```python
from build123d import *

# Parameters (mm, degrees)
F1_DEPTH  = 3.175
F2_W      = 17.018
F2_H      = 8.128
F3_DEPTH  = 1.5875
F5_DEPTH  = 1.5875
F6_W      = 10.05
F6_H      = 8.76
F7_DEPTH  = 3
F8_R      = 3.5
F9_DEPTH  = 3.5
F11_DEPTH = 1.5875


with BuildPart() as f1:
    # F0 (on Top) → F1 (new body)
    with BuildSketch(Plane.XY):
        with BuildLine():
            Line((-12.0608898944, 10.16), (-19.05, 10.16))
            Line((-19.05, 10.16), (-19.05, 0))
            Line((-19.05, 0), (0, 0))
            Line((0, 0), (0, 10.16))
            Line((0, 10.16), (-6.9891101056, 10.16))
            ThreePointArc((-6.9891101056, 10.16), (-7.425, 10.06), (-7.8608898944, 10.16))
            Line((-7.8608898944, 10.16), (-9.0891101056, 10.16))
            ThreePointArc((-9.0891101056, 10.16), (-9.525, 10.06), (-9.9608898944, 10.16))
            Line((-9.9608898944, 10.16), (-11.1891101056, 10.16))
            ThreePointArc((-11.1891101056, 10.16), (-11.625, 10.06), (-12.0608898944, 10.16))
        make_face()
        with BuildLine():
            ThreePointArc((-10.625, 11.06), (-12.1560885546, 11.9073163206), (-12.0608898944, 10.16))
            Line((-12.0608898944, 10.16), (-11.1891101056, 10.16))
            ThreePointArc((-11.1891101056, 10.16), (-10.7776836794, 10.5289114454), (-10.625, 11.06))
        make_face()
        with BuildLine():
            Line((-11.1891101056, 10.16), (-12.0608898944, 10.16))
            ThreePointArc((-12.0608898944, 10.16), (-11.625, 10.06), (-11.1891101056, 10.16))
        make_face()
        with BuildLine():
            ThreePointArc((-8.525, 11.06), (-10.0560885546, 11.9073163206), (-9.9608898944, 10.16))
            Line((-9.9608898944, 10.16), (-9.0891101056, 10.16))
            ThreePointArc((-9.0891101056, 10.16), (-8.6776836794, 10.5289114454), (-8.525, 11.06))
        make_face()
        with BuildLine():
            Line((-9.0891101056, 10.16), (-9.9608898944, 10.16))
            ThreePointArc((-9.9608898944, 10.16), (-9.525, 10.06), (-9.0891101056, 10.16))
        make_face()
        with BuildLine():
            ThreePointArc((-7.8608898944, 10.16), (-7.425, 10.06), (-6.9891101056, 10.16))
            Line((-6.9891101056, 10.16), (-7.8608898944, 10.16))
        make_face()
        with BuildLine():
            Line((-7.8608898944, 10.16), (-6.9891101056, 10.16))
            ThreePointArc((-6.9891101056, 10.16), (-6.5776836794, 10.5289114454), (-6.425, 11.06))
            ThreePointArc((-6.425, 11.06), (-7.9560885546, 11.9073163206), (-7.8608898944, 10.16))
        make_face()
    extrude(amount=F1_DEPTH)

    # F2 (on face) → F3 (cut)
    with BuildSketch(Plane.XY.offset(3.175)):
        with Locations((-9.525, 5.08)):
            Rectangle(F2_W, F2_H)
    extrude(amount=-F3_DEPTH, mode=Mode.SUBTRACT)

    # F4 (on face) → F5 (join, through all)
    with BuildSketch(Plane.XY.offset(1.5875)):
        Polygon((-9.525, 8.5074082457), (-9.525, 9.144), (-10.1615917543, 9.144), (-18.034, 1.6525917543), (-18.034, 1.016), (-17.3974082457, 1.016), (-9.825, 8.2219273099), align=None)
        Polygon((-8.8884082457, 9.144), (-9.525, 9.144), (-9.525, 8.5074082457), (-9.225, 8.2219273099), (-1.6525917543, 1.016), (-1.016, 1.016), (-1.016, 1.6525917543), align=None)
    extrude(amount=F5_DEPTH)

    # F6 (on face) → F7 (join)
    with BuildSketch(Plane(origin=(0, 0, 0), x_dir=(1, 0, 0), z_dir=(0, 0, -1))):
        with Locations((-9.525, -5.08)):
            Rectangle(F6_W, F6_H)
    extrude(amount=F7_DEPTH)

    # F8 (on face) → F9 (cut)
    with BuildSketch(Plane(origin=(0, 0, -3), x_dir=(1, 0, 0), z_dir=(0, 0, -1))):
        with Locations((-9.525, -5.08)):
            Circle(F8_R)
    extrude(amount=-F9_DEPTH, mode=Mode.SUBTRACT)

    # F10 (on face) → F11 (join, through all)
    with BuildSketch(Plane.XY.offset(1.5875)):
        Polygon((-9.525, 8.5074082457), (-9.975, 8.0791868419), (-9.975, 1.016), (-9.525, 1.016), (-9.075, 1.016), (-9.075, 8.0791868419), align=None)
    extrude(amount=F11_DEPTH)


solid = f1.part
```
Here's how the part is built. I have some questions about the finished solid (model axes, mm). A direction names the side the tool comes from. Give positions to 0.01 mm unless a question says otherwise; leave off trailing zeros. Write each loop counter-clockwise with the first axis right and the second up, starting at its lowest first coordinate (ties: lowest second). Pieces come first, ordered by that corner, then holes. Notation, with made-up numbers: (13.5, 3) -> (48.5, 3) arc R15 cw to (48.5, 29) -> close; hole circle Ø6 at (9, 12.25). An arc over 180 degrees is marked (long way). Use one line per item in the form item = value.
1) On a 3-axis mill with a long thin cutter (end or side, diameter ignored), from which of +Z, -Z, +X, -X, +Y, -Y can I reach the whole of each face in a straight line? I mean faces 4 (the face through (-14.55, 5, -1)), 5 (the face through (-12, 8, -3)), 6 (the face through (-5.42, 4.6, 2.37)), 7 (the face through (-4.5, 5, -1)), 8 (the face through (-10, 0.7, -1)). Say none if no direction works.
Verdict:
face_4 = -Z, -X, +Y, -Y
face_5 = -Z, +X, -X, +Y, -Y
face_6 = +Z
face_7 = -Z, +X, +Y, -Y
face_8 = -Z, +X, -X, -Y
2) Suppose I cut it at B-B (x = -3). Please give me the cut outline in (y, z) (1 decimal).
Verdict:
outline = (0, 0) -> (10.2, 0) -> (10.2, 3.2) -> (9.1, 3.2) -> (9.1, 1.6) -> (3.5, 1.6) -> (3.5, 3.2) -> (2.3, 3.2) -> (2.3, 1.6) -> (1, 1.6) -> (1, 3.2) -> (0, 3.2) -> close
3) If I drill on L1, parallel to X at y = 5.08, z = -1.7 (3 decimals); L2, parallel to Z at x = -13.5, y = 2.5; L3, parallel to Y at x = -13.25, z = -2, over which ranges is the centre line in solid material (lowest first)? Write a range as [from, to].
Verdict:
L1 = [-14.55, -13.025], [-6.025, -4.5]
L2 = [-3, 1.59]
L3 = [0.7, 9.46]
4) I'm going to push flat-ended pins straight in: pin 1 (1.6 mm diameter, centred on x = -16.5, z = 2, fed in from +Y); pin 2 (0.6 mm diameter, centred on x = -10.5, z = 2, fed in from +Y); pin 3 (2 mm diameter, centred on x = -5.5, y = 3, fed in from +Z). Where does each tip first touch, or does it pass through?
Verdict:
pin_1 = 10.16
pin_2 = 11.8
pin_3 = 1.59
5) We'd pull the mould along X, two halves only. Please class faces 1 (the face through (-10, 0, 2)), 2 (the face through (0, 5, 2)), 3 (the face through (-3, 7, 1.588)): +X half, -X half, draft (parallel to the pull), parting line (faces both ways), or undercut.
Verdict:
face_1 = draft
face_2 = +X half
face_3 = undercut
6) Suppose I cut it at A-A (z = -2.5). Please give me the cut outline in (x, y) (3 decimals).
Verdict:
outline = (-14.55, 0.7) -> (-4.5, 0.7) -> (-4.5, 9.46) -> (-14.55, 9.46) -> close; hole circle Ø7 at (-9.525, 5.08)
